from build123d import *

# Parameters (mm, degrees)
SKETCH1_W               = 14
SKETCH1_H               = 24
SKETCH1_W_2             = 3
SKETCH1_H_2             = 3
PCB_DEPTH               = 1.2
SOLDER_JOINTS_DEPTH     = 2
SOLDER_FILLETS_R        = 1.125
SKETCH2_W               = 3.205722041
SKETCH2_H               = 3.205722042
SKETCH2_W_2             = 3.205722042
SKETCH2_W_3             = 2.430144128
SKETCH2_H_2             = 4.007152552
TOP_COMPONENTS_DEPTH    = 1
SKETCH3_W               = 4.033005149
SKETCH3_H               = 4.058308378
SKETCH3_W_2             = 3.102311653
SKETCH3_H_2             = 2.921343474
SKETCH3_W_3             = 2.817933085
SKETCH3_W_4             = 2.869638279
SKETCH3_W_5             = 1.835534395
SKETCH3_H_3             = 3.12816425
BOTTOM_COMPONENTS_DEPTH = 1


with BuildPart() as part:
    # Sketch1 → PCB (new body)
    with BuildSketch(Plane(origin=(0, 0, 0), x_dir=(1, 0, 0), z_dir=(0, 1, 0))):
        Rectangle(SKETCH1_W, SKETCH1_H)
        with Locations((-5.5, 13.5)):
            Rectangle(SKETCH1_W_2, SKETCH1_H_2)
        with Locations((0, 13.5)):
            Rectangle(SKETCH1_W_2, SKETCH1_H_2)
        with Locations((5.5, 13.5)):
            Rectangle(SKETCH1_W_2, SKETCH1_H_2)
    extrude(amount=PCB_DEPTH)

    # Sketch5 → Solder joints (add)
    with BuildSketch(Plane(origin=(0, 1.2, 0), x_dir=(1, 0, 0), z_dir=(0, 1, 0))):
        with BuildLine():
            Line((-4.375, 13.25), (-4.375, 13.75))
            ThreePointArc((-4.375, 13.75), (-5.5, 14.875), (-6.625, 13.75))
            Line((-6.625, 13.75), (-6.625, 13.25))
            ThreePointArc((-6.625, 13.25), (-5.5, 12.125), (-4.375, 13.25))
        make_face()
        with BuildLine():
            Line((-1.125, 13.75), (-1.125, 13.25))
            ThreePointArc((-1.125, 13.25), (0, 12.125), (1.125, 13.25))
            Line((1.125, 13.25), (1.125, 13.75))
            ThreePointArc((1.125, 13.75), (0, 14.875), (-1.125, 13.75))
        make_face()
        with BuildLine():
            Line((4.375, 13.75), (4.375, 13.25))
            ThreePointArc((4.375, 13.25), (5.5, 12.125), (6.625, 13.25))
            Line((6.625, 13.25), (6.625, 13.75))
            ThreePointArc((6.625, 13.75), (5.5, 14.875), (4.375, 13.75))
        make_face()
        with BuildLine():
            Line((-6.625, -10.25), (-6.625, -10.75))
            ThreePointArc((-6.625, -10.75), (-5.5, -11.875), (-4.375, -10.75))
            Line((-4.375, -10.75), (-4.375, -10.25))
            ThreePointArc((-4.375, -10.25), (-5.5, -9.125), (-6.625, -10.25))
        make_face()
        with BuildLine():
            ThreePointArc((6.625, -10.75), (5.5, -11.875), (4.375, -10.75))
            Line((4.375, -10.75), (4.375, -10.25))
            ThreePointArc((4.375, -10.25), (5.5, -9.125), (6.625, -10.25))
            Line((6.625, -10.25), (6.625, -10.75))
        make_face()
    extrude(amount=SOLDER_JOINTS_DEPTH)

    # Solder fillets
    solder_fillets_edges = [part.edges().sort_by_distance(p)[0] for p in [
        (-6.625, 3.2, -13.5),
        (-4.375, 3.2, -13.5),
        (-5.5, 3.2, -14.875),
        (-5.5, 3.2, -12.125),
        (1.125, 3.2, -13.5),
        (-1.125, 3.2, -13.5),
        (0, 3.2, -12.125),
        (0, 3.2, -14.875),
        (6.625, 3.2, -13.5),
        (4.375, 3.2, -13.5),
        (5.5, 3.2, -12.125),
        (5.5, 3.2, -14.875),
        (-4.375, 3.2, 10.5),
        (-6.625, 3.2, 10.5),
        (-5.5, 3.2, 11.875),
        (-5.5, 3.2, 9.125),
        (5.5, 3.2, 11.875),
        (6.625, 3.2, 10.5),
        (5.5, 3.2, 9.125),
        (4.375, 3.2, 10.5),
    ]]
    fillet(solder_fillets_edges, radius=SOLDER_FILLETS_R - 0.0001)  # a hair under: the kernel refuses the full size

    # Sketch2 → Top components (add)
    with BuildSketch(Plane(origin=(0, 1.2, 0), x_dir=(1, 0, 0), z_dir=(0, 1, 0))):
        with Locations((-4.369088912, 8.144117457)):
            Rectangle(SKETCH2_W, SKETCH2_H)
        with Locations((0.232673374, 8.144117457)):
            Rectangle(SKETCH2_W_2, SKETCH2_H)
        with Locations((4.860288257, 8.144117457)):
            Rectangle(SKETCH2_W, SKETCH2_H)
        with Locations((-4.937846048, 1.758525971)):
            Rectangle(SKETCH2_W_2, SKETCH2_H)
        with Locations((-0.18096818, 1.758525971)):
            Rectangle(SKETCH2_W_2, SKETCH2_H)
        with Locations((4.524204494, 1.758525971)):
            Rectangle(SKETCH2_W_2, SKETCH2_H)
        with Locations((-2.119912963, -3.68344572)):
            Rectangle(SKETCH2_W_3, SKETCH2_H_2)
    extrude(amount=TOP_COMPONENTS_DEPTH)

    # Sketch3 → Bottom components (add)
    with BuildSketch(Plane.XZ):
        with Locations((-0.775577914, 2.029154189)):
            Rectangle(SKETCH3_W, SKETCH3_H)
        with Locations((-4.343236315, -5.442521059)):
            Rectangle(SKETCH3_W_2, SKETCH3_H_2)
        with Locations((0.090484089, -5.442521059)):
            Rectangle(SKETCH3_W_3, SKETCH3_H_2)
        with Locations((4.511278196, -5.442521059)):
            Rectangle(SKETCH3_W_4, SKETCH3_H_2)
        with Locations((4.433720405, 7.923271646)):
            Rectangle(SKETCH3_W_5, SKETCH3_H_3)
    extrude(amount=BOTTOM_COMPONENTS_DEPTH)


solid = part.part
Source: CAD feature listing. Evaluate the final solid. Frame: model axes, mm. A direction names the side the tool comes from. Round coordinates to 2 decimals unless told otherwise and drop trailing zeros. Order: outer loops, then holes, each group sorted by start corner. A loop starts at its lowest first (then second) coordinate and runs counter-clockwise, first axis right, second up. Notation, with made-up numbers: (39.5, 29.25) - (95.5, 29.25) arc R20 cw to (95.5, 59.25) - close; hole circle Ø10 at (-38, 79.5). An arc over 180 degrees is marked (long way). Use a Markdown table: item, result. Add a question column.
1. Line query: probe 1 along Z at (x, y) = (-5.5, 1.8) (3 decimals); probe 2 along Y at (x, z) = (-5, -13.25); probe 3 along Z at (x, y) = (5.75, -0.65). Output: solid intervals per line, ascending.
2. Set-up query: faces 5 (the flat face through (-4, 1, -13)), 6 (the flat face through (-0.8, -0.5, 0)), 7 (the flat face through (5, 2.2, -8)), 8 (the flat face through (4.4, -0.5, 9.487)), 9 (the flat face through (1.422, 2, -2)). Return all of +Z, -Z, +X, -X, +Y, -Y with unobstructed straight access to the full face (end or side cutting, diameter ignored); none if empty.
3. Mould query, pull axis X, two halves, no side actions, for faces 1 (the flat face through (-5, 2, -0.156)), 2 (the flat face through (1.499, -0.5, -5.5)), 3 (the flat face through (-1.784, 2, -2)), 4 (the cylindrical face through (6.304, 2.862, -13.504)). Classes: +X half, -X half, draft (parallel to the pull), parting line (faces both ways), or undercut.
4. Section query C-C (y = 0.7). Return the cut outline in (x, z).
5. Section query A-A (y = -0.5). Return the cut outline in (x, z), then the cut area to 3 significant figures.
6. First-contact query: pin 1 (0.5 mm diameter, centred on x = 4.5, y = -0.5, fed in from -Z); pin 2 (1 mm diameter, centred on x = -5.5, z = -2.5, fed in from +Y); pin 3 (4 mm diameter, centred on x = 0, z = 6.5, fed in from -Y). Flat tips, straight axial feed; report the tip coordinate or a pass-through.
7. Section query D-D (z = -6.25). Return the cut outline in (x, y).
8. Section query B-B (z = 4.5). Return the cut outline in (x, y), then the cut area to 3 significant figures.
Derived:
| question | item | result |
|---|---|---|
| 1 | probe 1 | -14.875 to -12.125, -9.747 to -6.541, -3.361 to -0.156, 9.125 to 11.875 |
| 1 | probe 2 | 0 to 3.08 |
| 1 | probe 3 | -6.9 to -3.98 |
| 2 | face 5 | -Z, +Y, -Y |
| 2 | face 6 | +X, -X, -Y |
| 2 | face 7 | +X, -X, +Y |
| 2 | face 8 | +Z, +X, -X, -Y |
| 2 | face 9 | +Z, +Y |
| 3 | face 1 | draft |
| 3 | face 2 | undercut |
| 3 | face 3 | undercut |
| 3 | face 4 | +X half |
| 4 | outline | (-7, -15) - (-4, -15) - (-4, -12) - (-1.5, -12) - (-1.5, -15) - (1.5, -15) - (1.5, -12) - (4, -12) - (4, -15) - (7, -15) - (7, 12) - (-7, 12) - close |
| 5 | outline | (-5.89, -6.9) - (-2.79, -6.9) - (-2.79, -3.98) - (-5.89, -3.98) - close; (-2.79, 0) - (1.24, 0) - (1.24, 4.06) - (-2.79, 4.06) - close; (-1.32, -6.9) - (1.5, -6.9) - (1.5, -3.98) - (-1.32, -3.98) - close; (3.08, -6.9) - (5.95, -6.9) - (5.95, -3.98) - (3.08, -3.98) - close; (3.52, 6.36) - (5.35, 6.36) - (5.35, 9.49) - (3.52, 9.49) - close |
| 5 | area | 47.8 mm2 |
| 6 | pin 1 | z = -6.9 |
| 6 | pin 2 | y = 2.2 |
| 6 | pin 3 | y = 0 |
| 7 | outline | (-7, 0) - (-5.89, 0) - (-5.89, -1) - (-2.79, -1) - (-2.79, 0) - (-1.32, 0) - (-1.32, -1) - (1.5, -1) - (1.5, 0) - (3.08, 0) - (3.08, -1) - (5.95, -1) - (5.95, 0) - (7, 0) - (7, 1.2) - (-7, 1.2) - close |
| 8 | outline | (-7, 0) - (7, 0) - (7, 1.2) - (-0.9, 1.2) - (-0.9, 2.2) - (-3.33, 2.2) - (-3.33, 1.2) - (-7, 1.2) - close |
| 8 | area | 19.2 mm2 |
